Geometry: see drawing. Coordinates: mm, zero at the bounding-box minimum. Give positions to 0.01 mm unless a question says otherwise; leave off trailing zeros. Loops run counter-clockwise (first coordinate to the right, second up) from the corner with the lowest first, then second, coordinate; pieces in that order, holes last. Notation, with made-up numbers: (-18, 73.25) -> (-8, 73.25) arc R32 ccw to (-8, 107.25) -> close; hole circle Ø4 at (34, 43.25). An arc over 180 degrees is marked (long way). Return JSON: item names as keys, results as strings. Group by question number.
(1) Cut plane D-D on z = 5.2. Return loops of the section in (x, y).
(2) Pin query (flat end, axial travel): pin 1 (12 mm diameter, centred on x = 11, y = 12, fed in from -Z); pin 2 (3 mm diameter, centred on y = 10.5, z = 4, fed in from -X) (1 decimal); pin 3 (6 mm diameter, centred on x = 19, y = 23.5, fed in from +Z); pin 4 (3 mm diameter, centred on y = 9.5, z = 4, fed in from -X). Return the tip coordinate at first contact, or that it passes through.
(3) Cut plane C-C on z = 1.05. Return loops of the section in (x, y).
(4) Ray query, line 1 (Y direction, x = 27.5, z = 1.5); line 2 (Z direction, x = 11, y = 44.5); line 3 (X direction, y = 45, z = 2.7). Return the intervals inside material, ascending. Write a range as from..to.
(5) Cut plane B-B on x = 27.5. Give the number of separate pieces and of enclosed holes in the cut face, then the cut area to 3 significant figures.
(6) Draft query along X for the marked faces 1, 2 and 3. Return one class per face: released by +X, released by -X, zero draft, split by the parting line, or undercut.
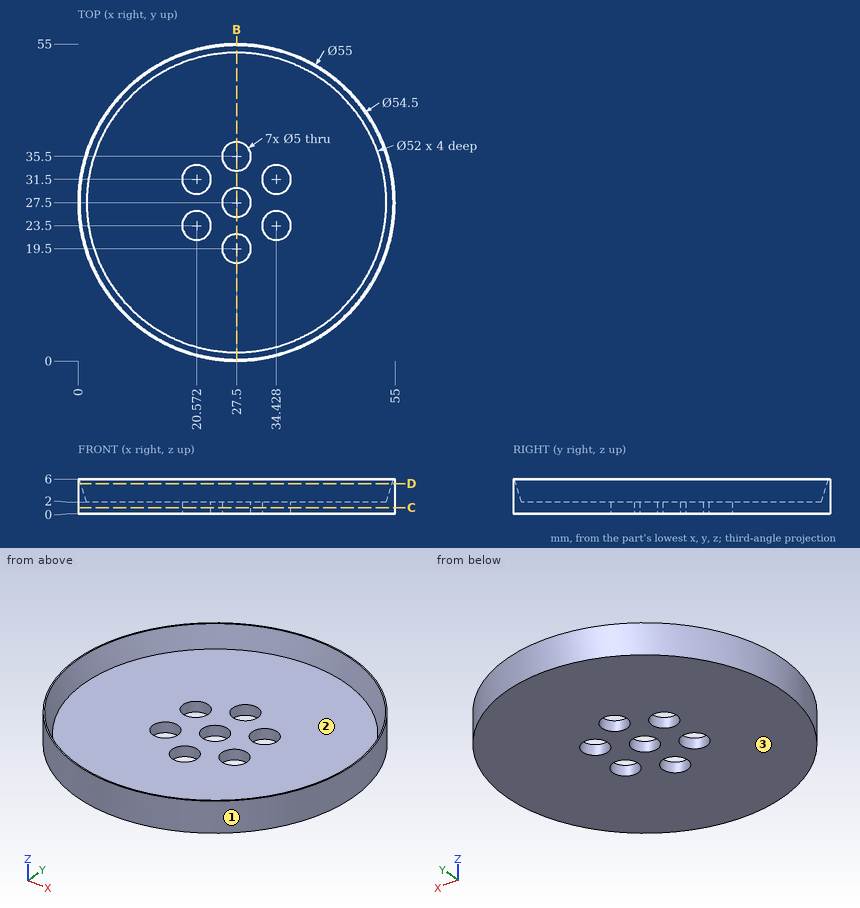
Answers:
{
 "1": {"outline": "circle Ø55 at (27.5, 27.5); hole circle Ø54 at (27.5, 27.5)"},
 "2": {"pin 1": "z = 0", "pin 2": "x = 4.8", "pin 3": "z = 2", "pin 4": "x = 5.5"},
 "3": {"outline": "circle Ø55 at (27.5, 27.5); hole circle Ø5 at (20.57, 23.5); hole circle Ø5 at (20.57, 31.5); hole circle Ø5 at (27.5, 19.5); hole circle Ø5 at (27.5, 27.5); hole circle Ø5 at (27.5, 35.5); hole circle Ø5 at (34.43, 23.5); hole circle Ø5 at (34.43, 31.5)"},
 "4": {"line 1": "0..17, 22..25, 30..33, 38..55", "line 2": "0..2", "line 3": "6.29..7.98, 47.02..48.71"},
 "5": {"separate pieces": "4", "enclosed holes": "0", "area": "87.0 mm²"},
 "6": {"face 1": "split by the parting line", "face 2": "undercut", "face 3": "zero draft"}
}
